from build123d import *

# Parameters (mm, degrees)
F1_DEPTH = 6
F2_SIZE2 = 4
F2_SIZE  = 19.5
F3_W     = 45
F3_H     = 7
F4_DEPTH = 6
F5_W     = 30
F5_H     = 6
F6_DEPTH = 14
F7_W     = 30
F7_H     = 14
F8_DEPTH = 6
F9_SIZE2 = 11.99999
F9_SIZE  = 13.99999


# Not quite as in the source:
# - a fillet or chamfer is up to 0.001 mm smaller than in the source, because OpenCascade refuses the exact size


with BuildPart() as f1:
    # F0 (on Front) → F1 (new body)
    with BuildSketch(Plane.XZ):
        with BuildLine():
            ThreePointArc((0, 44), (-15.9099025767, 37.4099025767), (-22.5, 21.5))
            Line((-22.5, 21.5), (0, 21.5))
            Line((0, 21.5), (0, 44))
        make_face()
        with BuildLine():
            ThreePointArc((0, -1), (-15.9099025767, 5.5900974233), (-22.5, 21.5))
            Line((-22.5, 21.5), (-22.5, -21.5))
            Line((-22.5, -21.5), (0, -21.5))
            Line((0, -21.5), (0, -1))
        make_face()
        with BuildLine():
            Line((0, 21.5), (-22.5, 21.5))
            ThreePointArc((-22.5, 21.5), (-15.9099025767, 5.5900974233), (0, -1))
            Line((0, -1), (0, 21.5))
        make_face()
        with BuildLine():
            Line((0, 44), (0, 21.5))
            Line((0, 21.5), (22.5, 21.5))
            ThreePointArc((22.5, 21.5), (15.9099025767, 37.4099025767), (0, 44))
        make_face()
        with BuildLine():
            Line((22.5, 21.5), (0, 21.5))
            Line((0, 21.5), (0, -1))
            ThreePointArc((0, -1), (15.9099025767, 5.5900974233), (22.5, 21.5))
        make_face()
        with BuildLine():
            ThreePointArc((22.5, 21.5), (15.9099025767, 5.5900974233), (0, -1))
            Line((0, -1), (0, -21.5))
            Line((0, -21.5), (22.5, -21.5))
            Line((22.5, -21.5), (22.5, 21.5))
        make_face()
    extrude(amount=F1_DEPTH)

    # F2
    f2_edges = [f1.edges().sort_by_distance(p)[0] for p in [
        (0, -6, 44),
    ]]
    f2_side = f1.faces().sort_by_distance((0, -6, 9.043566))[0]
    chamfer(f2_edges, length=F2_SIZE, length2=F2_SIZE2, reference=f2_side)

    # F3 (on face) → F4 (join)
    with BuildSketch(Plane(origin=(0, 0, 0), x_dir=(-1, 0, 0), z_dir=(0, 1, 0))):
        with Locations((0, -18)):
            Rectangle(F3_W, F3_H)
    extrude(amount=-F4_DEPTH)

    # F5 (on face) → F6 (join)
    with BuildSketch(Plane(origin=(0, 0, -21.5), x_dir=(1, 0, 0), z_dir=(0, 0, -1))):
        with Locations((0, 3)):
            Rectangle(F5_W, F5_H)
    extrude(amount=F6_DEPTH)

    # F7 (on face) → F8 (join)
    with BuildSketch(Plane(origin=(0, 0, 0), x_dir=(-1, 0, 0), z_dir=(0, 1, 0))):
        with Locations((0, -28.5)):
            Rectangle(F7_W, F7_H)
    extrude(amount=F8_DEPTH)

    # F9 (size 14 and 12 in the source; OpenCascade refuses exactly that, so slightly less here)
    f9_edges = [f1.edges().sort_by_distance(p)[0] for p in [
        (0, 6, -35.5),
    ]]
    f9_side = f1.faces().sort_by_distance((0, 6, -28.5))[0]
    chamfer(f9_edges, length=F9_SIZE, length2=F9_SIZE2, reference=f9_side)


solid = f1.part
Geometry check sheet. Reference: the model listing, model coordinates, mm. A direction names the side the tool comes from. Round coordinates to 2 decimals unless told otherwise and drop trailing zeros. Loops run counter-clockwise (first coordinate to the right, second up) from the corner with the lowest first, then second, coordinate; pieces in that order, holes last.
Item 1: Access from +Z, -Z, +X, -X, +Y, -Y to the whole of each face (thin tool, end or side, straight path). Record for faces 1 (the flat face through (0, 3, -21.5)), 2 (the flat face through (-12.89, -3.97, 3.75)), 3 (the flat face through (12.89, -3.97, 3.25)), 4 (the flat face through (15, -1, -27)), 5 (the flat face through (-19, -3, -21.5)).
Item 2: Cross-section at C-C on y = -1. Record the boundary of the cut face in (x, z), then the cut area to 3 significant figures.
Item 3: Gauge pin test, flat ends, axial feed: pin 1 (1.8 mm diameter, centred on x = 19, y = -3.5, fed in from -Z); pin 2 (22.5 mm diameter, centred on x = -1, z = -4.5, fed in from +Y); pin 3 (10 mm diameter, centred on x = -17, z = 16.5, fed in from -Y). Record the tip position at first contact, or that the pin passes through.
Item 4: Cross-section at B-B on z = -17. Record the boundary of the cut face in (x, y).
Item 5: Thickness scan on line 1 (X direction, y = -2, z = -26); line 2 (Z direction, x = -18, y = -4.5); line 3 (Y direction, x = -3, z = -5.5). Record the ranges inside material, lowest first.
Item 6: Cross-section at D-D on z = 11. Record the boundary of the cut face in (x, y).
Answer sheet:
1. face 1: +Z, +X, -X, +Y
1. face 2: +Z, -X, -Y
1. face 3: +Z, +X, -Y
1. face 4: -Z, +X, +Y, -Y
1. face 5: -Z, -X, +Y, -Y
2. outline: (-22.5, -21.5) - (-15, -21.5) - (-15, -29.67) - (15, -29.67) - (15, -21.5) - (22.5, -21.5) - (22.5, 21.5) arc R22.5 ccw to (-22.5, 21.5) - close
2. area: 2,980 mm2
3. pin 1: stops at z = -21.5
3. pin 2: stops at y = 0
3. pin 3: stops at y = -4.15
4. outline: (-22.5, -6) - (22.5, -6) - (22.5, 0) - (-22.5, 0) - close
5. line 1: x = -15 to 15
5. line 2: z = -21.5 to -14.5
5. line 3: y = -6 to 0
6. outline: (-22.5, -2) - (-3, -6) - (3, -6) - (22.5, -2) - (22.5, 0) - (-22.5, 0) - close
